```python
from build123d import *

# Parameters (mm, degrees)
SKETCH1_R             = 11.05
BOSS_EXTRUDE1_DEPTH   = 22.1
SKETCH4_R             = 9.525
BOSS_EXTRUDE3_DEPTH   = 30
F_3_0MM_DOWEL_HOLE1_D = 3


with BuildPart() as part:
    # Sketch1 → Boss-Extrude1 (new body)
    with BuildSketch(Plane(origin=(0, 0, 0), x_dir=(1, 0, 0), z_dir=(0, 1, 0))):
        with Locations(Location((0, 0, 0), (0, 0, 270))):
            Circle(SKETCH1_R)
    extrude(amount=BOSS_EXTRUDE1_DEPTH)

    # Sketch4 → Boss-Extrude3 (add)
    with BuildSketch(Plane.XY):
        with Locations(Location((0, 11.05, 0), (0, 0, 180))):
            Circle(SKETCH4_R)
    extrude(amount=BOSS_EXTRUDE3_DEPTH)

    # Ø3.0mm Dowel Hole1 (through all)
    with Locations(Plane(origin=(0, 0, 0), x_dir=(-1, 0, 0), z_dir=(0, -1, 0))):
        with Locations((7.07, 0), (0, 7.07), (-7.07, 0), (0, -7.07)):
            Hole(F_3_0MM_DOWEL_HOLE1_D / 2)


solid = part.part
```
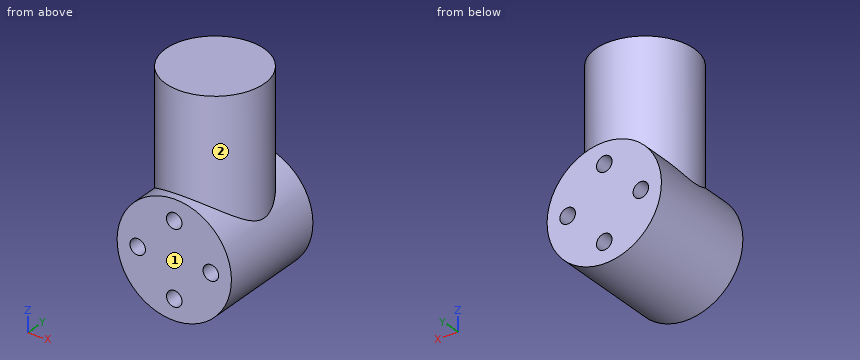
Can you work these out from the model? Positions are in its coordinate system, mm. Face numbers are marked on the shaded views. A direction names the side the tool comes from. Round coordinates to 2 decimals unless told otherwise and drop trailing zeros. Loops run counter-clockwise (first coordinate to the right, second up) from the corner with the lowest first, then second, coordinate; pieces in that order, holes last. Notation, with made-up numbers: M 81,82 L 129,82 A8 ccw 129,94 Z; hole C 2,54.25 d3. An arc over 180 degrees is marked long. Write item = value, one per line. Start each with the question number.
(1) Suppose I cut it at A-A on x = 0. Write out the boundary of the cut face in (y, z) (3 decimals).
(2) Suppose I cut it at D-D on x = -7.07. Write out the boundary of the cut face in (y, z), plus the area to 3 significant figures.
(3) I'm going to push flat-ended pins straight in: P1, Ø5, axis at x = -7.07, z = 0, coming from the -Y side; P2, Ø2.5, axis at x = 0, z = -7.07, coming from the +Y side; P3, Ø12, axis at x = -2, z = 25, coming from the -Y side (3 decimals); P4, Ø8, axis at y = 17, z = 10.5, coming from the -X side. Where does each tip first touch, or does it pass through?
(4) Which directions (+Z, -Z, +X, -X, +Y, -Y) give clear straight access to the entire face, cutting with the end or side of a thin tool? Please do the marked faces 1 and 2.
(5) Suppose I cut it at B-B on y = 11.05. Give the number of separate pieces and of enclosed holes in the cut face, plus the area to 3 significant figures.
(6) Suppose I cut it at C-C on z = 0. Write out the boundary of the cut face in (x, y), plus the area to 3 significant figures.
(7) I need wall thicknesses on line 1 along Z through (x, y) = (7.07, 9.5); line 2 along X through (y, z) = (8.25, -7.07); line 3 along X through (y, z) = (11.25, -7.5). Which ranges of each line are inside material? Lowest first, please.
Answer block:
q1.outline = M 0,-11.05 L 22.1,-11.05 L 22.1,-8.57 L 0,-8.57 Z; M 0,-5.57 L 22.1,-5.57 L 22.1,5.57 L 0,5.57 Z; M 0,8.57 L 22.1,8.57 L 22.1,11.05 L 20.575,11.05 L 20.575,30 L 1.525,30 L 1.525,11.05 L 0,11.05 Z
q2.outline = M 0,-8.49 L 22.1,-8.49 L 22.1,-1.5 L 0,-1.5 Z; M 0,1.5 L 22.1,1.5 L 22.1,8.49 L 17.43,8.49 L 17.43,30 L 4.67,30 L 4.67,8.49 L 0,8.49 Z
q2.area = 584 mm²
q3.P1 = 0
q3.P2 = through
q3.P3 = 1.525
q3.P4 = -9.32
q4.face_1 = +Z, -Z, +X, -X, -Y
q4.face_2 = +Z
q5.separate_pieces = 1
q5.enclosed_holes = 4
q5.area = 747 mm²
q6.outline = M -11.05,0 L -8.57,0 L -8.57,22.1 L -11.05,22.1 Z; M -5.57,0 L 5.57,0 L 5.57,22.1 L -5.57,22.1 Z; M 8.57,0 L 11.05,0 L 11.05,22.1 L 8.57,22.1 Z
q6.area = 356 mm²
q7.line_1 = -8.49 to -1.5, 1.5 to 30
q7.line_2 = -8.49 to -1.5, 1.5 to 8.49
q7.line_3 = -8.11 to -1.44, 1.44 to 8.11
